Model file for the job. Use its own axes, mm. A direction names the side the tool comes from. Give positions to 0.01 mm unless a question says otherwise; leave off trailing zeros. Loops run counter-clockwise (first coordinate to the right, second up) from the corner with the lowest first, then second, coordinate; pieces in that order, holes last. Notation, with made-up numbers: (36, -4.75) - (57, -4.75) arc R25 ccw to (57, 21.25) - close; hole circle Ø5 at (14.25, 74). An arc over 180 degrees is marked (long way). Answer as CSV lines item,"result". Start each with the question number.
Item 1: Saw through at B-B on x = 0. Give the cut face in (y, z).
Item 2: Saw through at C-C on y = 15. Give the cut face in (x, z), plus the area to 3 significant figures.
Item 3: Tool access for faces 1 (the flat face through (41, 5, 48.738)), 2 (the flat face through (-41, 5, 14.277)), 3 (the flat face through (0, 30, 32)), 4 (the flat face through (-41, 5, 46.738)), 5 (the flat face through (-41, 5, 48.738)): list every direction of +Z, -Z, +X, -X, +Y, -Y with a clear straight run to the whole face (end or side of a thin tool).
Item 4: Pin check, flat tips, straight feed: pin 1 (1.5 mm diameter, centred on x = 32.5, z = 11.5, fed in from -Y); pin 2 (11 mm diameter, centred on x = -43, y = 5, fed in from -Z); pin 3 (6.5 mm diameter, centred on x = -41.5, y = 6, fed in from +Z); pin 4 (3 mm diameter, centred on x = 0, y = 15, fed in from +Z). Stop position of each tip, or through.
Item 5: Saw through at A-A on z = 45.5. Give the cut face in (x, y).
Item 6: Pull direction Z, two halves, no side cores. Call faces 6 (the flat face through (41, 5, 14.277)), 7 (the flat face through (37, 0, 31)), 8 (the flat face through (-37.858, 5, 32)): pulls with the +Z half, pulls with the -Z half, needs draft (parallel to the pull), parting line crosses it, or undercut.
Item 7: Drill centre lines: L1, parallel to X at y = 3, z = 46.5; L2, parallel to Y at x = 0, z = 30.75; L3, parallel to Z at x = 40, y = 7. Where is each one in solid material? Low to high. Write a range as from..to.
Item 8: Saw through at D-D on y = 23. Give the cut face in (x, z).
from build123d import *

# Parameters (mm, degrees)
SKETCH4_W           = 6
SKETCH4_H           = 30.460968249
BOSS_EXTRUDE3_DEPTH = 10
SKETCH5_R           = 4.75
BOSS_EXTRUDE4_DEPTH = 20
CUT_EXTRUDE1_REACH  = 73.611
SKETCH6_R           = 2.5
CUT_EXTRUDE2_REACH  = 101.208


with BuildPart() as part:
    # Sketch4 → Boss-Extrude3 (new body)
    with BuildSketch(Plane(origin=(0, 0, 0), x_dir=(1, 0, 0), z_dir=(0, 1, 0))):
        with BuildLine():
            Line((35.857927804, -48.738130517), (45.857927804, -48.738130517))
            Line((45.857927804, -48.738130517), (45.857927804, -14.277162268))
            Line((45.857927804, -14.277162268), (35.857927804, -14.277162268))
            ThreePointArc((35.857927804, -14.277162268), (0, 9.842170723), (-35.857927804, -14.277162268))
            Line((-35.857927804, -14.277162268), (-45.857927804, -14.277162268))
            Line((-45.857927804, -14.277162268), (-45.857927804, -48.738130517))
            Line((-45.857927804, -48.738130517), (-35.857927804, -48.738130517))
            ThreePointArc((-35.857927804, -48.738130517), (0, -72.857463508), (35.857927804, -48.738130517))
        make_face()
        with Locations((40.857927804, -31.507646392)):
            Rectangle(SKETCH4_W, SKETCH4_H, mode=Mode.SUBTRACT)
        with Locations((-40.857927804, -31.507646392)):
            Rectangle(SKETCH4_W, SKETCH4_H, mode=Mode.SUBTRACT)
    extrude(amount=BOSS_EXTRUDE3_DEPTH)

    # Sketch5 → Boss-Extrude4 (add)
    with BuildSketch(Plane(origin=(0, 10, 0), x_dir=(1, 0, 0), z_dir=(0, 1, 0))):
        with Locations(Location((0, -31.507646393, 0), (0, 0, 90))):
            Circle(SKETCH5_R)
    extrude(amount=BOSS_EXTRUDE4_DEPTH)

    # Sketch6 → Cut-Extrude1 (cut, up to next)
    with BuildSketch(Plane(origin=(0, 0, 26.757646393), x_dir=(-1, 0, 0), z_dir=(0, 0, -1)), mode=Mode.PRIVATE) as cut_extrude1_sk1:
        with Locations((0, 15)):
            Circle(SKETCH6_R)
    cut_extrude1_tool1 = extrude(cut_extrude1_sk1.sketch, amount=-CUT_EXTRUDE1_REACH, mode=Mode.PRIVATE) & part.part
    add(cut_extrude1_tool1.solids().sort_by_distance((0, 15, 26.757646))[0], mode=Mode.SUBTRACT)

    # Sketch7 → Cut-Extrude2 (cut, up to next)
    with BuildSketch(Plane.XY.offset(72.857463508), mode=Mode.PRIVATE) as cut_extrude2_sk1:
        with BuildLine():
            Line((-35.857927804, 0), (35.857927804, 0))
            ThreePointArc((35.857927804, 0), (0, 2.127613267), (-35.857927804, 0))
        make_face()
    cut_extrude2_tool1 = extrude(cut_extrude2_sk1.sketch, amount=-CUT_EXTRUDE2_REACH, mode=Mode.PRIVATE) & part.part
    add(cut_extrude2_tool1.solids().sort_by_distance((0, 0.851302, 72.857464))[0], mode=Mode.SUBTRACT)


solid = part.part
Responses:
1,outline,"(2.13, -9.84) - (10, -9.84) - (10, 26.76) - (12.5, 26.76) - (12.5, 36.26) - (10, 36.26) - (10, 72.86) - (2.13, 72.86) - close; (17.5, 26.76) - (30, 26.76) - (30, 36.26) - (17.5, 36.26) - close"
2,outline,"(-2.5, 27.47) - (-2.5, 35.55) arc R4.75 ccw to start; (2.5, 27.47) arc R4.75 ccw to (2.5, 35.55) - close"
2,area,"25.7 mm2"
3,face 1,"+Z, +X, +Y, -Y"
3,face 2,"-Z, -X, +Y, -Y"
3,face 3,"+Z, -Z, +X, -X, +Y"
3,face 4,"+Y, -Y"
3,face 5,"+Z, -X, +Y, -Y"
4,pin 1,"y = 0.3"
4,pin 2,"z = 14.28"
4,pin 3,"z = 48.74"
4,pin 4,"through"
5,outline,"(-45.86, 0) - (-43.86, 0) - (-43.86, 10) - (-45.86, 10) - close; (-37.86, 0) - (-35.86, 0) arc R303.23 cw to (35.86, 0) - (37.86, 0) - (37.86, 10) - (-37.86, 10) - close; (43.86, 0) - (45.86, 0) - (45.86, 10) - (43.86, 10) - close"
6,face 6,"pulls with the -Z half"
6,face 7,"needs draft"
6,face 8,"undercut"
7,L1,"-45.86..-43.86, -37.86..37.86, 43.86..45.86"
7,L2,"2.13..12.5, 17.5..30"
7,L3,"14.28..16.28, 46.74..48.74"
8,outline,"circle Ø9.5 at (0, 31.51)"
